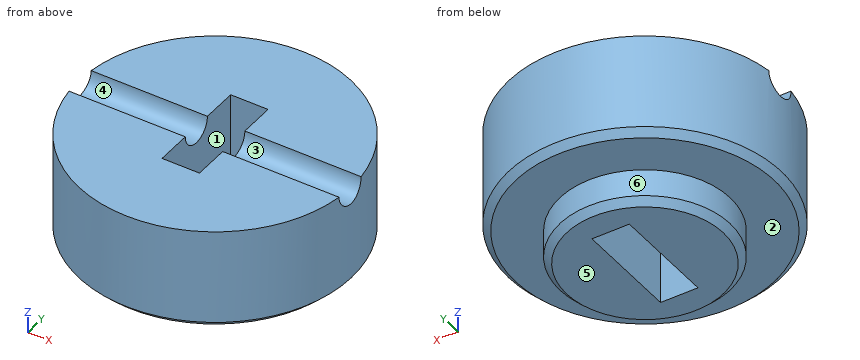
```python
from build123d import *

# Parameters (mm, degrees)
F0_R     = 4
F1_DEPTH = 3
F2_R     = 2.5
F3_DEPTH = 1
F4_R     = 0.5
F5_DEPTH = 9
F6_W     = 1.1
F6_H     = 1.05
F6_H_2   = 1
F7_DEPTH = 4.001
F8_SIZE  = 0.2


# Not quite as in the source:
# - a feature names something its author has since deleted; it is built from what else it names


with BuildPart() as f1:
    # F0 (on Top) → F1 (new body)
    with BuildSketch(Plane.XY):
        Circle(F0_R)
    extrude(amount=-F1_DEPTH)

    # F2 (on face) → F3 (join)
    with BuildSketch(Plane(origin=(0, 0, -3), x_dir=(1, 0, 0), z_dir=(0, 0, -1))):
        Circle(F2_R)
    extrude(amount=F3_DEPTH)

    # F4 (on Right) → F5 (cut, symmetric)
    with BuildSketch(Plane.YZ):
        Circle(F4_R)
    extrude(amount=F5_DEPTH, both=True, mode=Mode.SUBTRACT)

    # F6 (on face) → F7 (cut, through all)
    with BuildSketch(Plane.XY):
        with Locations((0, -1.025)):
            Rectangle(F6_W, F6_H)
        Rectangle(F6_W, F6_H_2)
        with Locations((0, 1.025)):
            Rectangle(F6_W, F6_H)
    extrude(amount=-F7_DEPTH, mode=Mode.SUBTRACT)

    # F8
    f8_edges = [f1.edges().sort_by_distance(p)[0] for p in [
        (-4, 0, -3),
        (-2.5, 0, -4),
    ]]
    chamfer(f8_edges, length=F8_SIZE)


solid = f1.part
```
Check sheet for the modelled part. Datum: model origin and axes. Units: mm. Face numbers are marked on the shaded views. A direction names the side the tool comes from. Give positions to 0.01 mm unless a question says otherwise; leave off trailing zeros. Write each loop counter-clockwise with the first axis right and the second up, starting at its lowest first coordinate (ties: lowest second). Pieces come first, ordered by that corner, then holes.
Item 1: Cross-section at A-A (y = 0). Enter the section's corners in (x, z), and give its area (3 significant figures).
Item 2: Cross-section at D-D (z = -1.15). Enter the section's corners in (x, y).
Item 3: Draft check along Y on the marked faces 4, 5 and 6. Enter one of: released by +Y, released by -Y, zero draft, split by the parting line, or undercut.
Item 4: Cross-section at C-C (z = -3.55). Enter the section's corners in (x, y).
Item 5: Cross-section at B-B (x = 0). Enter the section's corners in (y, z), and give its area (3 significant figures).
Item 6: Scan lines: L1, parallel to X at y = 1.25, z = -2.6; L2, parallel to Z at x = -1, y = 3.25; L3, parallel to Y at x = -0.5, z = -0.9. Record each from-to range of solid material in increasing order.
Item 7: Gauge pin test, flat end, axial feed: pin 1 (1.5 mm diameter, centred on x = -0.5, z = -3.5, fed in from -Y). Record the tip position at first contact, or that the pin passes through.
Item 8: Access from +Z, -Z, +X, -X, +Y, -Y to the whole of each face (thin tool, end or side, straight path). Record for the marked faces 1, 2 and 3.
Report:
1. outline: (-4, -2.8) - (-3.8, -3) - (-2.5, -3) - (-2.5, -3.8) - (-2.3, -4) - (-0.55, -4) - (-0.55, -0.5) - (-4, -0.5) - close; (0.55, -4) - (2.3, -4) - (2.5, -3.8) - (2.5, -3) - (3.8, -3) - (4, -2.8) - (4, -0.5) - (0.55, -0.5) - close
1. area: 21.1 mm2
2. outline: circle Ø8 at (0, 0); hole (-0.55, -1.55) - (0.55, -1.55) - (0.55, 1.55) - (-0.55, 1.55) - close
3. face 4: undercut
3. face 5: zero draft
3. face 6: split by the parting line
4. outline: circle Ø5 at (0, 0); hole (-0.55, -1.55) - (0.55, -1.55) - (0.55, 1.55) - (-0.55, 1.55) - close
5. outline: (-4, -2.8) - (-3.8, -3) - (-2.5, -3) - (-2.5, -3.8) - (-2.3, -4) - (-1.55, -4) - (-1.55, 0) - (-4, 0) - close; (1.55, -4) - (2.3, -4) - (2.5, -3.8) - (2.5, -3) - (3.8, -3) - (4, -2.8) - (4, 0) - (1.55, 0) - close
5. area: 16.5 mm2
6. L1: x = -3.8 to -0.55, 0.55 to 3.8
6. L2: z = -3 to 0
6. L3: y = -3.97 to -1.55, 1.55 to 3.97
7. pin 1: stops at y = -3.99
8. face 1: +Z, -Z
8. face 2: -Z
8. face 3: +Z, +X, -X
